Source: CAD feature listing. Evaluate the final solid. Frame: model axes, mm. Round coordinates to 2 decimals unless told otherwise and drop trailing zeros. Loops run counter-clockwise (first coordinate to the right, second up) from the corner with the lowest first, then second, coordinate; pieces in that order, holes last. Notation, with made-up numbers: (79, -16) -> (134, -16) arc R20 ccw to (134, 9) -> close; hole circle Ø10 at (84, 42.25). An arc over 180 degrees is marked (long way). Write item = value, one per line.
from build123d import *

# Parameters (mm, degrees)
SKETCH1_W                    = 717.55
SKETCH1_H                    = 787.4
BOSS_EXTRUDE1_DEPTH          = 3.175
SWERVE_CUTOUT_DEPTH          = 533.662436492
SKETCH2_W                    = 228.6
SKETCH2_H                    = 447.675
INTAKE_CUTOUT_DEPTH          = 3.175
F_8_0_199_DIAMETER_HOLE1_D   = 5.0546
F_30_0_1285_DIAMETER_HOLE1_D = 3.2639
FILLET1_R                    = 6.35
CHAMFER1_SIZE                = 2.54


with BuildPart() as part:
    # Sketch1 → Boss-Extrude1 (new body)
    with BuildSketch(Plane(origin=(0, 0, 0), x_dir=(1, 0, 0), z_dir=(0, 1, 0))):
        Rectangle(SKETCH1_W, SKETCH1_H)
    extrude(amount=BOSS_EXTRUDE1_DEPTH)

    # Sketch8 → Swerve Cutout (cut, through all)
    with BuildSketch(Plane(origin=(0, 3.175, 0), x_dir=(1, 0, 0), z_dir=(0, 1, 0))):
        with BuildLine():
            Line((358.775, 285.755663772), (358.775, 393.7))
            Line((358.775, 393.7), (250.830663772, 393.7))
            Line((250.830663772, 393.7), (250.830663772, 368.3))
            Line((250.830663772, 368.3), (239.222863772, 368.3))
            ThreePointArc((239.222863772, 368.3), (251.852591334, 286.777591334), (333.375, 274.147863772))
            Line((333.375, 274.147863772), (333.375, 285.755663772))
            Line((333.375, 285.755663772), (358.775, 285.755663772))
        make_face()
        with BuildLine():
            Line((333.375, -285.755663772), (333.375, -274.147863772))
            ThreePointArc((333.375, -274.147863772), (251.852591334, -286.777591334), (239.222863772, -368.3))
            Line((239.222863772, -368.3), (250.830663772, -368.3))
            Line((250.830663772, -368.3), (250.830663772, -393.7))
            Line((250.830663772, -393.7), (358.775, -393.7))
            Line((358.775, -393.7), (358.775, -285.755663772))
            Line((358.775, -285.755663772), (333.375, -285.755663772))
        make_face()
        with BuildLine():
            Line((-358.775, -285.755663772), (-358.775, -393.7))
            Line((-358.775, -393.7), (-250.830663772, -393.7))
            Line((-250.830663772, -393.7), (-250.830663772, -368.3))
            Line((-250.830663772, -368.3), (-239.222863772, -368.3))
            ThreePointArc((-239.222863772, -368.3), (-251.852591334, -286.777591334), (-333.375, -274.147863772))
            Line((-333.375, -274.147863772), (-333.375, -285.755663772))
            Line((-333.375, -285.755663772), (-358.775, -285.755663772))
        make_face()
        with BuildLine():
            Line((-333.375, 285.755663772), (-333.375, 274.147863772))
            ThreePointArc((-333.375, 274.147863772), (-251.852591334, 286.777591334), (-239.222863772, 368.3))
            Line((-239.222863772, 368.3), (-250.830663772, 368.3))
            Line((-250.830663772, 368.3), (-250.830663772, 393.7))
            Line((-250.830663772, 393.7), (-358.775, 393.7))
            Line((-358.775, 393.7), (-358.775, 285.755663772))
            Line((-358.775, 285.755663772), (-333.375, 285.755663772))
        make_face()
    extrude(amount=-SWERVE_CUTOUT_DEPTH, mode=Mode.SUBTRACT)

    # Sketch2 → Intake Cutout (cut)
    with BuildSketch(Plane(origin=(0, 3.175, 0), x_dir=(1, 0, 0), z_dir=(0, 1, 0))):
        with Locations((244.475, 0)):
            Rectangle(SKETCH2_W, SKETCH2_H)
    extrude(amount=-INTAKE_CUTOUT_DEPTH, mode=Mode.SUBTRACT)

    # #8 (0.199) Diameter Hole1 (through all)
    with Locations(Plane(origin=(0, 3.175, 0), x_dir=(1, 0, 0), z_dir=(0, 1, 0))):
        with Locations((244.480663772, 381), (219.080663772, 381), (193.680663772, 381), (346.075, 279.405663772), (346.075, 254.005663772), (346.075, 228.605663772), (346.075, -228.605663772), (346.075, -254.005663772), (346.075, -279.405663772), (193.680663772, -381), (219.080663772, -381), (244.480663772, -381), (-244.480663772, -381), (-219.080663772, -381), (-193.680663772, -381), (-346.075, -279.405663772), (-346.075, -254.005663772), (-346.075, -228.605663772), (-346.075, 228.605663772), (-346.075, 254.005663772), (-346.075, 279.405663772), (-193.680663772, 381), (-219.080663772, 381), (-244.480663772, 381)):
            Hole(F_8_0_199_DIAMETER_HOLE1_D / 2)

    # #30 (0.1285) Diameter Hole1 (through all)
    with Locations(Plane(origin=(0, 3.175, 0), x_dir=(1, 0, 0), z_dir=(0, 1, 0))):
        with Locations((-139.7, 384.175), (-114.3, 377.825), (-88.9, 384.175), (-63.5, 377.825), (-38.1, 384.175), (-12.7, 377.825), (12.7, 384.175), (38.1, 377.825), (63.5, 384.175), (88.9, 377.825), (114.3, 384.175), (139.7, 377.825), (165.1, 384.175), (-165.1, 377.825), (-165.1, -377.825), (165.1, -384.175), (139.7, -377.825), (114.3, -384.175), (88.9, -377.825), (63.5, -384.175), (38.1, -377.825), (12.7, -384.175), (-12.7, -377.825), (-38.1, -384.175), (-63.5, -377.825), (-88.9, -384.175), (-114.3, -377.825), (-139.7, -384.175), (-342.9, -203.2), (-349.25, -177.8), (-342.9, -152.4), (-349.25, -127), (-342.9, -101.6), (-349.25, -76.2), (-342.9, -50.8), (-349.25, -25.4), (-342.9, 0), (-349.25, 25.4), (-342.9, 50.8), (-349.25, 76.2), (-342.9, 101.6), (-349.25, 127), (-342.9, 152.4), (-349.25, 177.8), (-342.9, 203.2)):
            Hole(F_30_0_1285_DIAMETER_HOLE1_D / 2)

    # Fillet1
    fillet1_edges = [part.edges().sort_by_distance(p)[0] for p in [
        (239.222863772, 1.5875, 368.3),
        (333.375, 1.5875, 274.147863772),
        (-239.222863772, 1.5875, 368.3),
        (-333.375, 1.5875, 274.147863772),
        (-239.222863772, 1.5875, -368.3),
        (-333.375, 1.5875, -274.147863772),
        (239.222863772, 1.5875, -368.3),
        (333.375, 1.5875, -274.147863772),
    ]]
    fillet(fillet1_edges, radius=FILLET1_R)

    # Chamfer1
    chamfer1_edges = [part.edges().sort_by_distance(p)[0] for p in [
        (358.775, 1.5875, -223.8375),
        (358.775, 1.5875, 223.8375),
        (358.775, 1.5875, 285.755663772),
        (250.830663772, 1.5875, 393.7),
        (-250.830663772, 1.5875, 393.7),
        (-358.775, 1.5875, 285.755663772),
        (-358.775, 1.5875, -285.755663772),
        (-250.830663772, 1.5875, -393.7),
        (250.830663772, 1.5875, -393.7),
        (358.775, 1.5875, -285.755663772),
    ]]
    chamfer(chamfer1_edges, length=CHAMFER1_SIZE)


solid = part.part
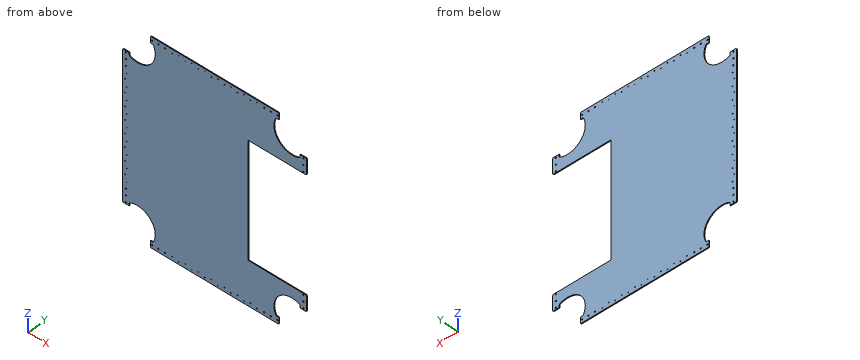
1. Contact query for flat-ended pins moving along their axis: pin 1 Ø1 at (x, z) = (127.5, -193.5) entering from -Y; pin 2 Ø2.5 at (x, z) = (-342.9, 50.8) entering from +Y; pin 3 Ø1 at (y, z) = (1, 216) entering from +X (3 decimals). Output: stop coordinate, or through.
Evaluation:
pin_1 = 0
pin_2 = through
pin_3 = 130.175
2. Section query B-B (y = 0.65). Give the number of separate pieces and of enclosed holes in the cut face, then the cut area to 3 significant figures.
Evaluation:
separate_pieces = 1
enclosed_holes = 69
area = 406,000 mm²
3. Line query: probe 1 along Z at (x, y) = (272.5, 1.1); probe 2 along Z at (x, y) = (-297, 1.15); probe 3 along X at (y, z) = (1.5, 50.8) (3 decimals). Output: solid intervals per line, ascending. Write a range as from..to.
Evaluation:
probe_1 = -272.51..-223.84, 223.84..272.51
probe_2 = -266.45..266.45
probe_3 = -358.775..-344.532, -341.268..130.175
4. Section query A-A (x = 311). Return the cut outline in (y, z) (1 decimal), then the cut area to 3 significant figures.
Evaluation:
outline = (0, -267) -> (3.2, -267) -> (3.2, -223.8) -> (0, -223.8) -> close; (0, 223.8) -> (3.2, 223.8) -> (3.2, 267) -> (0, 267) -> close
area = 274 mm²
